Could you check a few things on this model? Use its own coordinates, in mm. Face numbers are marked on the shaded views. Round coordinates to 2 decimals unless told otherwise and drop trailing zeros. Loops run counter-clockwise (first coordinate to the right, second up) from the corner with the lowest first, then second, coordinate; pieces in that order, holes last. Notation, with made-up numbers: (29.25, 73) - (63.25, 73) arc R10 ccw to (63.25, 84) - close; hole circle Ø3 at (51, 39.5). An arc over 180 degrees is marked (long way). Answer as CSV lines item,"result". Start each with the question number.
1) Please list where these lines run through material, in increasing order: line 1 along Z through (x, y) = (-45, 2); line 2 along X through (y, z) = (-2, 35); line 3 along X through (y, z) = (-2.5, 35).
2) We'd pull the mould along X, two halves only. Please class the marked faces 1, 2, 3 and 4: pulls with the +X half, pulls with the -X half, needs draft (parallel to the pull), parting line crosses it, or undercut.
3) Suppose I cut it at A-A, the plane z = 35. Write out the boundary of the cut face in (x, y), then the cut area to 3 significant figures.
4) Suppose I cut it at C-C, the plane y = -1.5. Write out the boundary of the cut face in (x, z).
5) Suppose I cut it at D-D, the plane z = 64.5. Write out the boundary of the cut face in (x, y).
6) Suppose I cut it at B-B, the plane x = 45. Write out the boundary of the cut face in (y, z), then the cut area to 3 significant figures.
7) I'm going to push a flat-ended pin straight in: pin 1 Ø1 at (y, z) = (0, 28) entering from -X. Where does the tip first touch, or does it pass through?
Autodesk Inventor part; units mm, degrees
ref_plane "YZ Plane" through (0, 0, 0) normal (1, 0, 0) x (0, 1, 0)
ref_plane "XZ Plane" through (0, 0, 0) normal (0, 1, 0) x (-1, 0, 0)
ref_plane "XY Plane" through (0, 0, 0) normal (0, 0, 1) x (1, 0, 0)
sketch "Schizzo1" plane through (0, 0, 0) normal (0, 0, 1) x (1, 0, 0)
  line L0 (-75, 4.5) -> (75, 4.5)
  line L1 (75, 4.5) -> (75, -4.5)
  line L2 (75, -4.5) -> (-75, -4.5)
  line L3 (-75, -4.5) -> (-75, 4.5)
  line L4 (-75, 4.5) -> (75, -4.5) construction
  line L5 (75, 4.5) -> (-75, -4.5) construction
  arc A0 (-75, 4.5) -> (-66, -4.5) centre (-66, 4.5) ccw
  arc A1 (66, -4.5) -> (75, 4.5) centre (66, 4.5) ccw
  point P0 (0, 0)
  dimension "d0" = 150
  dimension "d1" = 9
  dimension "d3" = 9
  dimension "d4" = 9
extrude "Estrusione1" add sketch "Schizzo1" along normal blind 70 contours L0 A1 L2 A0
sketch "Schizzo2" plane through (-66, -4.5, 0) normal (0, -1, 0) x (1, 0, 0)
  line L0 (141, 0) -> (141, 70)
  line L1 (-9, 0) -> (-9, 70)
  point P0 (66, 0)
  point P1 (21, 35)
  point P2 (111, 35)
  point P3 (141, 35)
  dimension "d7" = 30
  dimension "d8" = 30
  dimension "d16" = 90
hole "Foro1" at (-45, -4.5, 35) at (45, -4.5, 35) direction (0, 1, 0) diameter 10 end through all
properties part number "Spessore plastica"
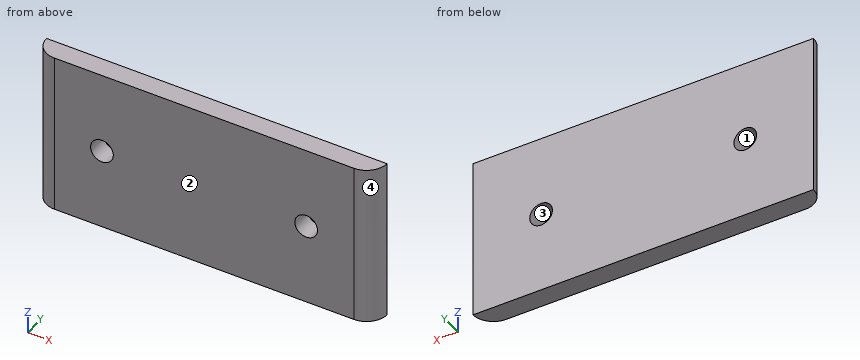
Filled sheet:
1,line 1,"0 to 30, 40 to 70"
1,line 2,"-72.22 to -50, -40 to 40, 50 to 72.22"
1,line 3,"-71.66 to -50, -40 to 40, 50 to 71.66"
2,face 1,"undercut"
2,face 2,"needs draft"
2,face 3,"undercut"
2,face 4,"pulls with the +X half"
3,outline,"(-75, 4.5) arc R9 ccw to (-66, -4.5) - (-50, -4.5) - (-50, 4.5) - close; (-40, -4.5) - (40, -4.5) - (40, 4.5) - (-40, 4.5) - close; (50, -4.5) - (66, -4.5) arc R9 ccw to (75, 4.5) - (50, 4.5) - close"
3,area,"1,140 mm²"
4,outline,"(-72.71, 0) - (72.71, 0) - (72.71, 70) - (-72.71, 70) - close; hole circle Ø10 at (-45, 35); hole circle Ø10 at (45, 35)"
5,outline,"(-75, 4.5) arc R9 ccw to (-66, -4.5) - (66, -4.5) arc R9 ccw to (75, 4.5) - close"
6,outline,"(-4.5, 0) - (4.5, 0) - (4.5, 30) - (-4.5, 30) - close; (-4.5, 40) - (4.5, 40) - (4.5, 70) - (-4.5, 70) - close"
6,area,"540 mm²"
7,pin 1,"x = -74.06"
